Autodesk Inventor part; units mm, degrees
ref_plane "YZ Plane" through (0, 0, 0) normal (1, 0, 0) x (0, 1, 0)
ref_plane "XZ Plane" through (0, 0, 0) normal (0, 1, 0) x (-1, 0, 0)
ref_plane "XY Plane" through (0, 0, 0) normal (0, 0, 1) x (1, 0, 0)
sketch "Sketch1" plane through (0, 0, 0) normal (0, 0, 1) x (1, 0, 0)
  line L0 (-1.4564, 16.2472) -> (-1.4564, 9.9656)
  line L1 (-1.4564, 9.9656) -> (-7.738, 9.9656)
  line L2 (-7.738, 8.9656) -> (-1.4564, 8.9656)
  line L3 (-1.4564, 8.9656) -> (-1.4564, 2.684)
  line L4 (-0.4564, 2.684) -> (-0.4564, 8.9656)
  line L5 (-0.4564, 8.9656) -> (5.8252, 8.9656)
  line L6 (5.8252, 9.9656) -> (-0.4564, 9.9656)
  line L7 (-0.4564, 9.9656) -> (-0.4564, 16.2472)
  circle A0 centre (-0.9564, 9.4656) radius 6.8
extrude "Extrusion1" add sketch "Sketch1" against normal blind 83.6 contours A0 L7 L6 L5 L4 L3 L2 L1 L0
extrude "Extrusion2" add sketch "Sketch1" against normal blind 1 contours L0 L1 A0 | A0 L6 L7 | L2 L3 A0 | A0 L4 L5
properties part number "seringa inside"
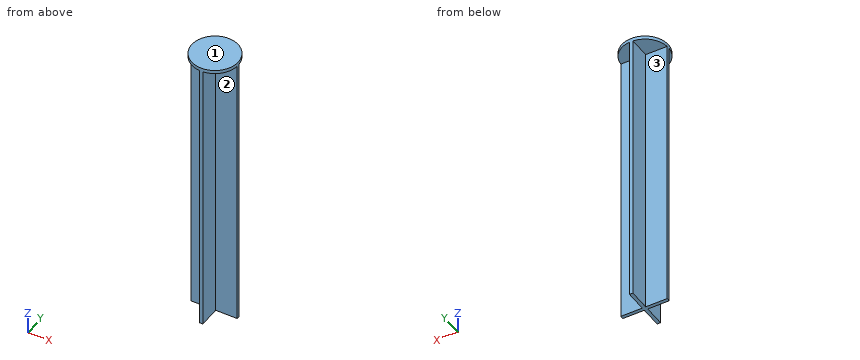
Verification items for the finished model (mm, model axes). Face numbers are marked on the shaded views. A direction names the side the tool comes from. Give positions to 0.01 mm unless a question says otherwise; leave off trailing zeros. Write each loop counter-clockwise with the first axis right and the second up, starting at its lowest first coordinate (ties: lowest second). Pieces come first, ordered by that corner, then holes.
(1) Gauge pin test, flat ends, axial feed: pin 1 (7 mm diameter, centred on x = -3, z = -28, fed in from -Y); pin 2 (1.5 mm diameter, centred on x = 1, y = 6, fed in from -Z); pin 3 (5 mm diameter, centred on x = -4.5, z = -45, fed in from +Y); pin 4 (7 mm diameter, centred on y = 13.5, z = -28, fed in from -X). Record the tip position at first contact, or that the pin passes through.
(2) Cross-section at A-A (z = -43). Enter the section's corners in (x, y).
(3) Cross-section at C-C (y = 15). Enter the section's corners in (x, z).
(4) Material ranges on line 1 (X direction, y = 10.75, z = -18.5); line 2 (Z direction, x = 5.25, y = 12); line 3 (Y direction, x = -2.5, z = -16), recorded low to high.
(5) Access from +Z, -Z, +X, -X, +Y, -Y to the whole of each face (thin tool, end or side, straight path). Record for the marked faces 1, 2 and 3.
(6) Cross-section at B-B (x = 4.25). Enter the section's corners in (y, z), plus the area to 3 significant figures.
Worked out:
1. pin 1: stops at y = 2.67
1. pin 2: stops at z = -1
1. pin 3: stops at y = 9.97
1. pin 4: stops at x = -1.46
2. outline: (-7.74, 8.97) - (-1.46, 8.97) - (-1.46, 2.68) arc R6.8 ccw to (-0.46, 2.68) - (-0.46, 8.97) - (5.83, 8.97) arc R6.8 ccw to (5.83, 9.97) - (-0.46, 9.97) - (-0.46, 16.25) arc R6.8 ccw to (-1.46, 16.25) - (-1.46, 9.97) - (-7.74, 9.97) arc R6.8 ccw to start
3. outline: (-4.91, -1) - (-1.46, -1) - (-1.46, -83.6) - (-0.46, -83.6) - (-0.46, -1) - (2.99, -1) - (2.99, 0) - (-4.91, 0) - close
4. line 1: x = -1.46 to -0.46
4. line 2: z = -1 to 0
4. line 3: y = 8.97 to 9.97
5. face 1: +Z, +X, -X, +Y, -Y
5. face 2: -Z, +X, -Y
5. face 3: -Z, -X, +Y
6. outline: (5.09, -1) - (8.97, -1) - (8.97, -83.6) - (9.97, -83.6) - (9.97, -1) - (13.84, -1) - (13.84, 0) - (5.09, 0) - close
6. area: 91.3 mm2
